Check sheet for the modelled part. Datum: model origin and axes. Units: mm. Give positions to 0.01 mm unless a question says otherwise; leave off trailing zeros. Loops run counter-clockwise (first coordinate to the right, second up) from the corner with the lowest first, then second, coordinate; pieces in that order, holes last. Notation, with made-up numbers: (50.25, -26.75) - (89.25, -26.75) arc R22 cw to (89.25, -7.75) - close; hole circle Ø1 at (33, -10.75). An arc over 180 degrees is marked (long way). Use one line per item in the form item = value.
from build123d import *

# Parameters (mm, degrees)
F0_R         = 50.8
F1_DEPTH     = 127
F2_T         = -10.16
F5_DEPTH     = 8.89
F6_T4_ANGLE  = 254.7462790776
F6_S5_R      = 50.8
F6_T6_DEPTH  = 89
F6_T11_ANGLE = 254.7462790776
F6_S12_R     = 50.8
F6_T13_DEPTH = 89
F6_T18_ANGLE = 254.7462790776
F6_S19_R     = 50.8
F6_T20_DEPTH = 89
F7_T4_ANGLE  = 254.3575983754
F7_S5_R      = 50.8
F7_T6_DEPTH  = 89
F7_T10_ANGLE = 254.3575983754


# Not quite as in the source:
# - a fillet or chamfer that OpenCascade refuses, or shapes differently, is made with other operations: its cross-section is extruded or revolved along the edge and cut away or added


with BuildPart() as f1:
    # F0 (on Top) → F1 (new body)
    with BuildSketch(Plane.XY):
        Circle(F0_R)
    extrude(amount=F1_DEPTH)

    # F2
    f2_openings = [f1.faces().sort_by_distance(p)[0] for p in [
        (0, 0, 127),
    ]]
    offset(amount=F2_T, openings=f2_openings)

    # F3: fillet of radius 10.4245741623 on 1 edges, made by hand

    # F3_s1 → F3_t2 (revolve, cut)
    with BuildSketch(Plane.XZ):
        with BuildLine():
            ThreePointArc((50.8, 127), (43.6003320895, 123.8559286261), (40.64, 116.5787838052))
            Line((40.64, 116.5787838052), (40.64, 127))
            Line((40.64, 127), (50.8, 127))
        make_face()
    revolve(axis=Axis((0, 0, 127), (0, 0, 1)), mode=Mode.SUBTRACT)

    # F4 (on Right) → F5 (join, symmetric)
    with BuildSketch(Plane.YZ):
        with BuildLine():
            ThreePointArc((40.9011468769, 118.0027031276), (96.7316605485, 61.0144931984), (45.3319139779, 0))
            ThreePointArc((45.3319139779, 0), (127.3418829144, 62.1638462438), (40.9011468769, 118.0027031276))
        make_face()
    extrude(amount=F5_DEPTH, both=True)

    # F6: fillet of radius 9.525 on 1 edges, made by hand


with BuildPart() as f6_tool2:
    # F6_s3 → F6_t4 (revolve)
    with BuildSketch(Plane(origin=(0, 8.968139316, -7.4168504874), x_dir=(1, 0, 0), z_dir=(0, -0.7706077503, 0.6373097325))):
        with BuildLine():
            ThreePointArc((-8.89, 33.9367221949), (-6.1001920908, 27.2015301041), (0.635, 24.4117221949))
            Line((0.635, 24.4117221949), (-8.89, 24.4117221949))
            Line((-8.89, 24.4117221949), (-8.89, 33.9367221949))
        make_face()
    revolve(axis=Axis((-8.89, 64.5634606481, 59.8066411912), (1, 0, 0)), revolution_arc=F6_T4_ANGLE)

    # F6_s5 → F6_t6 (intersect, symmetric)
    with BuildSketch(Plane.XY.offset(59.8)):
        Circle(F6_S5_R)
    extrude(amount=F6_T6_DEPTH, both=True, mode=Mode.INTERSECT)

    split(bisect_by=Plane.XY, keep=Keep.BOTTOM)


with BuildPart() as f1_1:
    add(f1.part)

    # F6_t1: cut F6_tool2
    add(f6_tool2.part, mode=Mode.SUBTRACT)


with BuildPart() as f6_tool9:
    # F6_s10 → F6_t11 (revolve)
    with BuildSketch(Plane(origin=(0, 8.968139316, -7.4168504874), x_dir=(1, 0, 0), z_dir=(0, -0.7706077503, 0.6373097325))):
        with BuildLine():
            ThreePointArc((-8.89, 33.9367221949), (-6.1001920908, 27.2015301041), (0.635, 24.4117221949))
            Line((0.635, 24.4117221949), (-8.89, 24.4117221949))
            Line((-8.89, 24.4117221949), (-8.89, 33.9367221949))
        make_face()
    revolve(axis=Axis((-8.89, 64.5634606481, 59.8066411912), (1, 0, 0)), revolution_arc=F6_T11_ANGLE)

    # F6_s12 → F6_t13 (cut, symmetric)
    with BuildSketch(Plane.XY.offset(59.8)):
        Circle(F6_S12_R)
    extrude(amount=F6_T13_DEPTH, both=True, mode=Mode.SUBTRACT)

    split(bisect_by=Plane.XY, keep=Keep.TOP)


with BuildPart() as f1_2:
    add(f1_1.part)

    # F6_t8: cut F6_tool9
    add(f6_tool9.part, mode=Mode.SUBTRACT)


with BuildPart() as f6_tool16:
    # F6_s17 → F6_t18 (revolve)
    with BuildSketch(Plane(origin=(0, 8.968139316, -7.4168504874), x_dir=(1, 0, 0), z_dir=(0, -0.7706077503, 0.6373097325))):
        with BuildLine():
            ThreePointArc((-8.89, 33.9367221949), (-6.1001920908, 27.2015301041), (0.635, 24.4117221949))
            Line((0.635, 24.4117221949), (-8.89, 24.4117221949))
            Line((-8.89, 24.4117221949), (-8.89, 33.9367221949))
        make_face()
    revolve(axis=Axis((-8.89, 64.5634606481, 59.8066411912), (1, 0, 0)), revolution_arc=F6_T18_ANGLE)

    # F6_s19 → F6_t20 (cut, symmetric)
    with BuildSketch(Plane.XY.offset(59.8)):
        Circle(F6_S19_R)
    extrude(amount=F6_T20_DEPTH, both=True, mode=Mode.SUBTRACT)

    split(bisect_by=Plane.XY, keep=Keep.BOTTOM)


with BuildPart() as f1_3:
    add(f1_2.part)

    # F6_t15: cut F6_tool16
    add(f6_tool16.part, mode=Mode.SUBTRACT)

    # F7: fillet of radius 9.525 on 1 edges, made by hand


with BuildPart() as f7_tool2:
    # F7_s3 → F7_t4 (revolve)
    with BuildSketch(Plane(origin=(0, 9.2218448194, -7.5741443116), x_dir=(1, 0, 0), z_dir=(0, -0.7727649908, 0.6346922632))):
        with BuildLine():
            ThreePointArc((0.635, 24.3717466269), (6.5351595171, 27.541577675), (8.89, 33.8117002814))
            Line((8.89, 33.8117002814), (8.89, 24.3717466269))
            Line((8.89, 24.3717466269), (0.635, 24.3717466269))
        make_face()
    revolve(axis=Axis((8.89, 64.5634606481, 59.8066411912), (1, 0, 0)), revolution_arc=F7_T4_ANGLE)

    # F7_s5 → F7_t6 (cut, symmetric)
    with BuildSketch(Plane.XY.offset(59.8)):
        Circle(F7_S5_R)
    extrude(amount=F7_T6_DEPTH, both=True, mode=Mode.SUBTRACT)


with BuildPart() as f1_4:
    add(f1_3.part)

    # F7_t1: cut F7_tool2
    add(f7_tool2.part, mode=Mode.SUBTRACT)


with BuildPart() as f7_tool8:
    # F7_s9 → F7_t10 (revolve)
    with BuildSketch(Plane(origin=(0, 9.2218448194, -7.5741443116), x_dir=(1, 0, 0), z_dir=(0, -0.7727649908, 0.6346922632))):
        with BuildLine():
            ThreePointArc((0.635, 24.3717466269), (6.5351595171, 27.541577675), (8.89, 33.8117002814))
            Line((8.89, 33.8117002814), (8.89, 24.3717466269))
            Line((8.89, 24.3717466269), (0.635, 24.3717466269))
        make_face()
    revolve(axis=Axis((8.89, 64.5634606481, 59.8066411912), (1, 0, 0)), revolution_arc=F7_T10_ANGLE)

    split(bisect_by=Plane.XY, keep=Keep.BOTTOM)


with BuildPart() as f1_5:
    add(f1_4.part)

    # F7_t7: cut F7_tool8
    add(f7_tool8.part, mode=Mode.SUBTRACT)


solid = f1_5.part
Item 1: Gauge pin test, flat ends, axial feed: P1, Ø12, axis at x = -12, y = -28.5, coming from the +Z side; P2, Ø12, axis at y = 18.5, z = 83.5, coming from the +X side; P3, Ø2, axis at y = -5, z = 52.5, coming from the +X side; P4, Ø17, axis at y = 76.5, z = 82, coming from the -X side. Record the tip position at first contact, or that the pin passes through.
Answer block:
P1 = 10.16
P2 = 49.24
P3 = 50.64
P4 = through
Item 2: Mould release check, pull along X, two halves, no side actions. Record for faces 1 (the face through (-1, 1, 10.16)), 2 (the face through (-11.012, -49.592, 62.611)), 3 (the face through (-8.89, 100, 64)), 4 (the face through (-5.291, 40.294, 62.624)): released by +X, released by -X, zero draft, split by the parting line, or undercut.
Answer block:
face_1 = undercut
face_2 = split by the parting line
face_3 = released by -X
face_4 = undercut
Item 3: Section check A-A on y = 0. Record the boundary of the cut face in (x, z).
Answer block:
outline = (-50.8, 0) - (50.8, 0) - (50.8, 127) arc R10.42 ccw to (40.64, 116.58) - (40.64, 10.16) - (-40.64, 10.16) - (-40.64, 116.58) arc R10.42 ccw to (-50.8, 127) - close
Item 4: Section check B-B on z = 73.5. Give the number of separate pieces and of enclosed holes in the cut face, then the cut area to 3 significant figures.
Answer block:
separate_pieces = 2
enclosed_holes = 1
area = 3,430 mm2
Item 5: Thickness scan on L1, parallel to X at y = 0, z = 46; L2, parallel to Y at x = 0, z = 76; L3, parallel to Y at x = 0, z = 89. Record the ranges inside material, lowest first.
Answer block:
L1 = -50.8 to -40.64, 40.64 to 50.8
L2 = -50.8 to -40.64, 40.64 to 50.8, 94.22 to 125.24
L3 = -50.8 to -40.64, 40.64 to 50.8, 88.5 to 120.17
